Build history of the part. All positions in model axes, mm. A direction names the side the tool comes from. Round coordinates to 2 decimals unless told otherwise and drop trailing zeros. Order: outer loops, then holes, each group sorted by start corner. A loop starts at its lowest first (then second) coordinate and runs counter-clockwise, first axis right, second up. Notation, with made-up numbers: (-17, 41) -> (13, 41) arc R7 ccw to (13, 45) -> close; hole circle Ø1 at (83, 10). An arc over 180 degrees is marked (long way). Answer as a JSON object with one key per item and string values.
from build123d import *

# Parameters (mm, degrees)
SKETCH1_W           = 88
SKETCH1_H           = 175
BOSS_EXTRUDE1_DEPTH = 1.5
SKETCH2_W           = 50
SKETCH2_H           = 39
CUT_EXTRUDE1_DEPTH  = 1.5
SKETCH3_R           = 2
BOSS_EXTRUDE2_DEPTH = 6


with BuildPart() as part:
    # Sketch1 → Boss-Extrude1 (new body)
    with BuildSketch(Plane(origin=(0, 0, 0), x_dir=(1, 0, 0), z_dir=(0, 1, 0))):
        Rectangle(SKETCH1_W, SKETCH1_H)
    extrude(amount=BOSS_EXTRUDE1_DEPTH)

    # Sketch2 → Cut-Extrude1 (cut)
    with BuildSketch(Plane(origin=(0, 1.5, 0), x_dir=(1, 0, 0), z_dir=(0, 1, 0))):
        with Locations((19, 42)):
            Rectangle(SKETCH2_W, SKETCH2_H)
    extrude(amount=-CUT_EXTRUDE1_DEPTH, mode=Mode.SUBTRACT)

    # Sketch3 → Boss-Extrude2 (add)
    with BuildSketch(Plane(origin=(0, 1.5, 0), x_dir=(1, 0, 0), z_dir=(0, 1, 0))):
        with Locations((37, 65)):
            Circle(SKETCH3_R)
        with Locations((25, 65)):
            Circle(SKETCH3_R)
        with Locations((13, 65)):
            Circle(SKETCH3_R)
    extrude(amount=BOSS_EXTRUDE2_DEPTH)


solid = part.part
1) Flat gauge pin, fed straight in: pin 1 Ø0.8 at (y, z) = (0.5, -49) entering from +X. Where does the tip first touch, or does it go through?
Checked values:
{"pin 1": "stops at x = -6"}
2) Cut at C-C, the plane z = -65. Give the cut face in (x, y), plus the area to 3 significant figures.
Checked values:
{"outline": "(-44, 0) -> (44, 0) -> (44, 1.5) -> (39, 1.5) -> (39, 7.5) -> (35, 7.5) -> (35, 1.5) -> (27, 1.5) -> (27, 7.5) -> (23, 7.5) -> (23, 1.5) -> (15, 1.5) -> (15, 7.5) -> (11, 7.5) -> (11, 1.5) -> (-44, 1.5) -> close", "area": "204 mm²"}
3) Cut at B-B, the plane y = 5.25. Give the cut face in (x, z).
Checked values:
{"outline": "circle Ø4 at (13, -65); circle Ø4 at (25, -65); circle Ø4 at (37, -65)"}
4) Cut at A-A, the plane x = 37. Give the cut face in (y, z), plus the area to 3 significant figures.
Checked values:
{"outline": "(0, -87.5) -> (1.5, -87.5) -> (1.5, -67) -> (7.5, -67) -> (7.5, -63) -> (1.5, -63) -> (1.5, -61.5) -> (0, -61.5) -> close; (0, -22.5) -> (1.5, -22.5) -> (1.5, 87.5) -> (0, 87.5) -> close", "area": "228 mm²"}
5) Which spindle directions (+Z, -Z, +X, -X, +Y, -Y) get a long thin tool onto all of the face, cutting with end or side? Do faces 4 (the face through (-1, 0, -1)), 5 (the face through (37, 4, -67)). Say none if no direction does.
Checked values:
{"face 4": "+Z, -Z, +X, -X, -Y", "face 5": "+Y"}
6) Cut at D-D, the plane z = 40.5. Give the cut face in (x, y), plus the area to 3 significant figures.
Checked values:
{"outline": "(-44, 0) -> (44, 0) -> (44, 1.5) -> (-44, 1.5) -> close", "area": "132 mm²"}
7) Probe L1, parallel to Z at x = 5.5, y = 1; L2, parallel to Y at x = -36, z = 71.5; L3, parallel to Z at x = 12.5, y = 3.5. List the from-to ranges inside material, lowest first. Write a range as from..to.
Checked values:
{"L1": "z = -87.5..-61.5, -22.5..87.5", "L2": "y = 0..1.5", "L3": "z = -66.94..-63.06"}
8) Pull direction X, two halves, no side cores. Call faces 1 (the face through (13, 4, -67)), 2 (the face through (25, 4, -67)), 3 (the face through (37, 7.5, -65)): pulls with the +X half, pulls with the -X half, needs draft (parallel to the pull), parting line crosses it, or undercut.
Checked values:
{"face 1": "undercut", "face 2": "undercut", "face 3": "needs draft"}
